Here's the drawing with two shaded views (mm, measured from the low corner). I have some questions. Coordinates: 2 decimals unless noted, no trailing zeros. Write each loop counter-clockwise with the first axis right and the second up, starting at its lowest first coordinate (ties: lowest second). Pieces come first, ordered by that corner, then holes.
Item 1: If we section it at C-C (y = 131): Please give me the cut outline in (x, z).
Item 2: I'm going to push flat-ended pins straight in: pin 1 Ø1.5 at (x, z) = (45, 2) entering from -Y; pin 2 Ø2.5 at (y, z) = (167, 4) entering from -X; pin 3 Ø3 at (y, z) = (154.5, 4) entering from +X; pin 4 Ø2.5 at (x, y) = (67.31, 106.68) entering from +Z. Where does each tip first touch, or does it pass through?
Item 3: If I drill on line 1 (X direction, y = 106.68, z = 3.95); line 2 (Y direction, x = 21.59, z = 1.7); line 3 (Y direction, x = 43.5, z = 4.6) (1 decimal), over which ranges is the centre line in solid material (lowest first)?
Item 4: If we section it at B-B (x = 49): Please give me the cut outline in (y, z), then the cut area to 3 significant figures.
Item 5: If we section it at D-D (z = 3.35): Count the separate pieces of the cut face and the enclosed holes in it, then the cut area to 3 significant figures.
Item 6: If we section it at A-A (y = 83.5): Please give me the cut outline in (x, z), then the cut area to 3 significant figures.
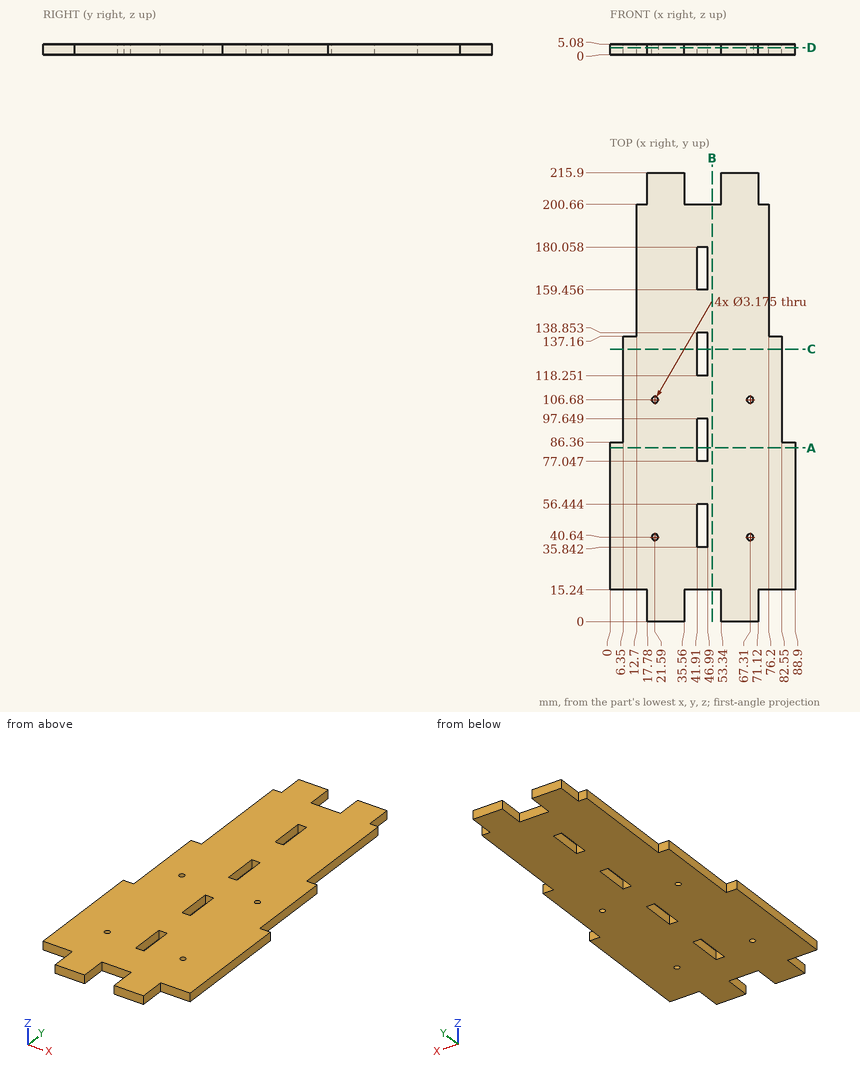
Answer list:
1. outline: (6.35, 0) - (41.91, 0) - (41.91, 5.08) - (6.35, 5.08) - close; (46.99, 0) - (82.55, 0) - (82.55, 5.08) - (46.99, 5.08) - close
2. pin 1: stops at y = 15.24
2. pin 2: stops at x = 12.7
2. pin 3: stops at x = 76.2
2. pin 4: passes through
3. line 1: x = 6.35 to 20, 23.18 to 65.72, 68.9 to 82.55
3. line 2: y = 0 to 39.05, 42.23 to 105.09, 108.27 to 215.9
3. line 3: y = 15.2 to 35.8, 56.4 to 77, 97.6 to 118.3, 138.9 to 159.5, 180.1 to 200.7
4. outline: (15.24, 0) - (200.66, 0) - (200.66, 5.08) - (15.24, 5.08) - close
4. area: 942 mm2
5. separate pieces: 1
5. enclosed holes: 8
5. area: 14,900 mm2
6. outline: (0, 0) - (41.91, 0) - (41.91, 5.08) - (0, 5.08) - close; (46.99, 0) - (88.9, 0) - (88.9, 5.08) - (46.99, 5.08) - close
6. area: 426 mm2
